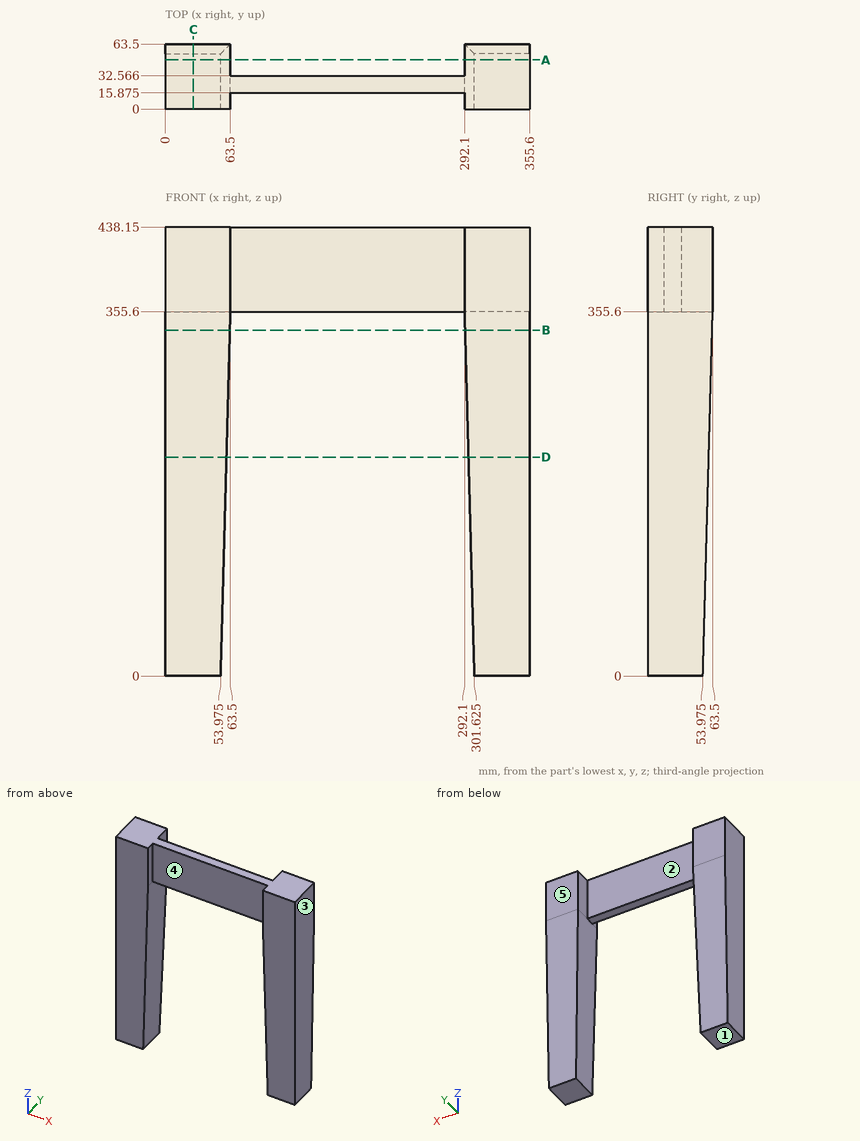
Geometry check sheet. Reference: drawing and pictorial views, mm from the part's lowest x, y, z. A direction names the side the tool comes from. Give positions to 0.01 mm unless a question says otherwise; leave off trailing zeros. Order: outer loops, then holes, each group sorted by start corner. A loop starts at its lowest first (then second) coordinate and runs counter-clockwise, first axis right, second up. Notation, with made-up numbers: M 76.5,-11 L 98.5,-11 A9 cw 98.5,-4 Z; hole C 88.5,72.25 d6. An arc over 180 degrees is marked long. Answer as a JSON object with one key per item and string values. Group by question number.
1) Cross-section at B-B (z = 337.5). Enter the section's corners in (x, y) (3 decimals), then the cut area to 3 significant figures.
2) Depth check by flat-ended pin: pin 1 Ø25 at (x, z) = (189.5, 386.5) entering from -Y (3 decimals); pin 2 Ø8.5 at (x, y) = (168.5, 27) entering from -Z; pin 3 Ø2 at (x, z) = (61, 304.5) entering from +Y. Enter the tip coordinate at first touch or a pass-through.
3) Access from +Z, -Z, +X, -X, +Y, -Y to the whole of each face (thin tool, end or side, straight path). Record for the marked faces 4 and 5.
4) Cross-section at D-D (z = 213.5). Enter the section's corners in (x, y).
5) Mould release check, pull along X, two halves, no side actions. Record for the marked faces 1, 2 and 3: released by +X, released by -X, zero draft, split by the parting line, or undercut.
6) Cross-section at C-C (x = 27.5). Enter the section's corners in (y, z) (3 decimals).
7) Scan lines: line 1 along Z through (x, y) = (168, 32); line 2 along X through (y, z) = (30.5, 331.5); line 3 along X through (y, z) = (25, 254.5). Record each from-to range of solid material in increasing order. Write a range as [from, to].
8) Cross-section at A-A (y = 48). Enter the section's corners in (x, z) (3 decimals), then the cut area to 3 significant figures.
Result sheet:
{
 "1": {"outline": "M 0,0 L 63.015,0 L 63.015,63.015 L 0,63.015 Z; M 292.585,0 L 355.6,0 L 355.6,63.015 L 292.585,63.015 Z", "area": "7,940 mm2"},
 "2": {"pin 1": "stops at y = 15.875", "pin 2": "stops at z = 355.6", "pin 3": "stops at y = 62.16"},
 "3": {"face 4": "+Z, -Z, -Y", "face 5": "+Z, -Z, +X, -X, +Y"},
 "4": {"outline": "M 0,0 L 59.69,0 L 59.69,59.69 L 0,59.69 Z; M 295.91,0 L 355.6,0 L 355.6,59.69 L 295.91,59.69 Z"},
 "5": {"face 1": "zero draft", "face 2": "undercut", "face 3": "released by +X"},
 "6": {"outline": "M 0,0 L 53.975,0 L 63.5,355.6 L 63.5,438.15 L 0,438.15 Z"},
 "7": {"line 1": "z = [355.6, 438.15]", "line 2": "x = [0, 62.85], [292.75, 355.6]", "line 3": "x = [0, 60.79], [294.81, 355.6]"},
 "8": {"outline": "M 0,0 L 53.975,0 L 63.5,355.6 L 63.5,438.15 L 0,438.15 Z; M 292.1,355.6 L 301.625,0 L 355.6,0 L 355.6,438.15 L 292.1,438.15 Z", "area": "52,300 mm2"}
}
